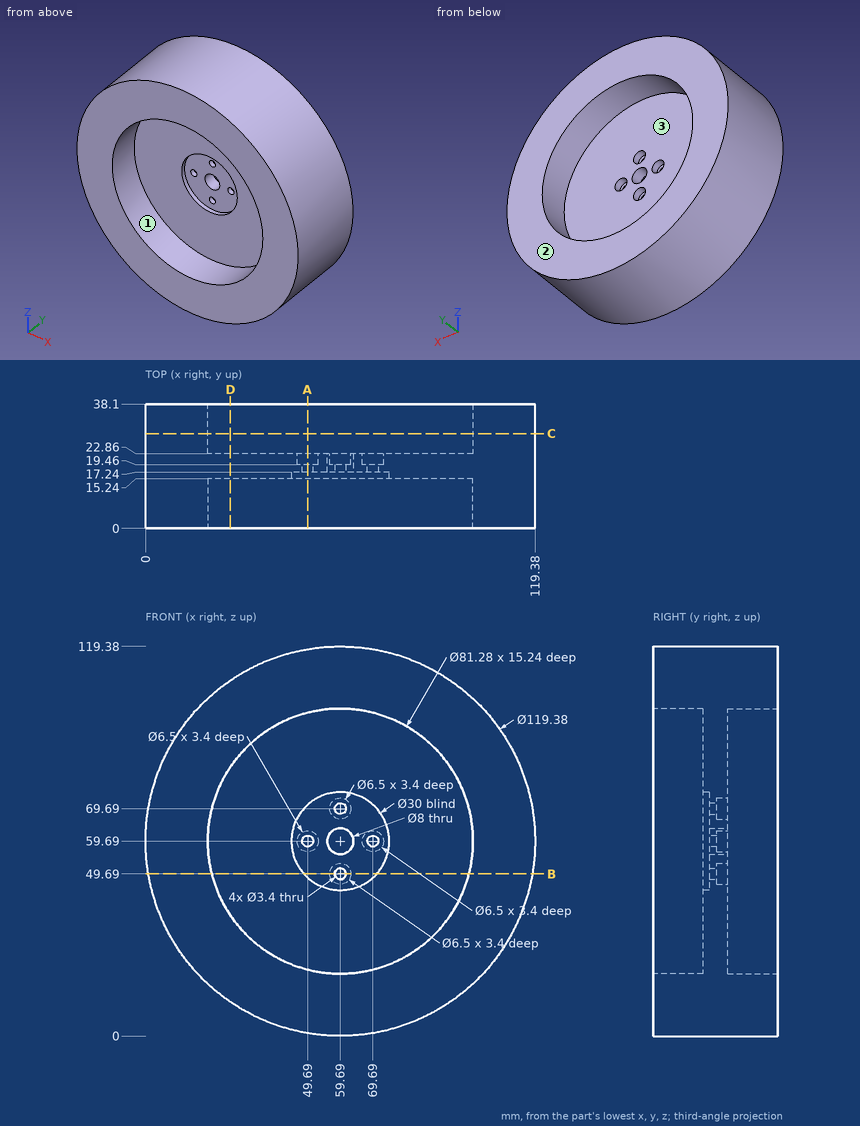
Geometry check sheet. Reference: drawing and pictorial views, mm from the part's lowest x, y, z. A direction names the side the tool comes from. Coordinates: 2 decimals unless noted, no trailing zeros. Order: outer loops, then holes, each group sorted by start corner. A loop starts at its lowest first (then second) coordinate and runs counter-clockwise, first axis right, second up. Notation, with made-up numbers: (52.25, 24) -> (91.25, 24) arc R4 ccw to (91.25, 28) -> close; hole circle Ø10 at (27, -37.75). An arc over 180 degrees is marked (long way). Use CSV: the item, a comma, the result in double quotes. Start each with the question number.
Q1. Section check B-B, the plane z = 49.69. Record the cut outline in (x, y).
Q2. Section check A-A, the plane x = 49.69. Record the cut outline in (y, z), and give its area (3 significant figures).
Q3. Depth check by flat-ended pin: P1, Ø1, axis at y = 12.5, z = 99, coming from the -X side; P2, Ø5, axis at x = 58, z = 51, coming from the +Y side; P3, Ø15, axis at x = 64.5, z = 54.5, coming from the -Y side. Enter the tip coordinate at first touch or a pass-through.
Q4. Section check C-C, the plane y = 29. Record the cut outline in (x, z).
Q5. Tool access check on the marked faces 1, 2 and 3. Record the directions out of +Z, -Z, +X, -X, +Y, -Y that give a thin tool (end or side, any length) a straight path to the whole face; none if there is none.
Q6. Section check D-D, the plane x = 26. Record the cut outline in (y, z).
Q7. Thickness scan on line 1 along Z through (x, y) = (59.69, 21.6); line 2 along X through (y, z) = (20, 59); line 3 along Z through (x, y) = (59.5, 31.5). Record the ranges inside material, lowest first.
Returned:
1,outline,"(0.84, 0) -> (20.3, 0) -> (20.3, 15.24) -> (48.51, 15.24) -> (48.51, 17.24) -> (57.99, 17.24) -> (57.99, 19.46) -> (56.44, 19.46) -> (56.44, 22.86) -> (20.3, 22.86) -> (20.3, 38.1) -> (0.84, 38.1) -> close; (61.39, 17.24) -> (70.87, 17.24) -> (70.87, 15.24) -> (99.08, 15.24) -> (99.08, 0) -> (118.54, 0) -> (118.54, 38.1) -> (99.08, 38.1) -> (99.08, 22.86) -> (62.94, 22.86) -> (62.94, 19.46) -> (61.39, 19.46) -> close"
2,outline,"(0, 0.84) -> (38.1, 0.84) -> (38.1, 20.3) -> (22.86, 20.3) -> (22.86, 56.44) -> (19.46, 56.44) -> (19.46, 57.99) -> (17.24, 57.99) -> (17.24, 48.51) -> (15.24, 48.51) -> (15.24, 20.3) -> (0, 20.3) -> close; (0, 99.08) -> (15.24, 99.08) -> (15.24, 70.87) -> (17.24, 70.87) -> (17.24, 61.39) -> (19.46, 61.39) -> (19.46, 62.94) -> (22.86, 62.94) -> (22.86, 99.08) -> (38.1, 99.08) -> (38.1, 118.54) -> (0, 118.54) -> close"
2,area,"2,010 mm^2"
3,P1,"stops at x = 14.34"
3,P2,"stops at y = 22.86"
3,P3,"stops at y = 17.24"
4,outline,"circle Ø119.38 at (59.69, 59.69); hole circle Ø81.28 at (59.69, 59.69)"
5,face 1,"-Y"
5,face 2,"+Z, -Z, +X, -X, +Y"
5,face 3,"+Y"
6,outline,"(0, 10.42) -> (38.1, 10.42) -> (38.1, 36.96) -> (22.86, 36.96) -> (22.86, 82.42) -> (38.1, 82.42) -> (38.1, 108.96) -> (0, 108.96) -> (0, 82.42) -> (15.24, 82.42) -> (15.24, 36.96) -> (0, 36.96) -> close"
7,line 1,"z = 0 to 46.44, 52.94 to 55.69, 63.69 to 66.44, 72.94 to 119.38"
7,line 2,"x = 0 to 46.51, 52.87 to 55.75, 63.63 to 66.51, 72.87 to 119.38"
7,line 3,"z = 0 to 19.05, 100.33 to 119.38"
